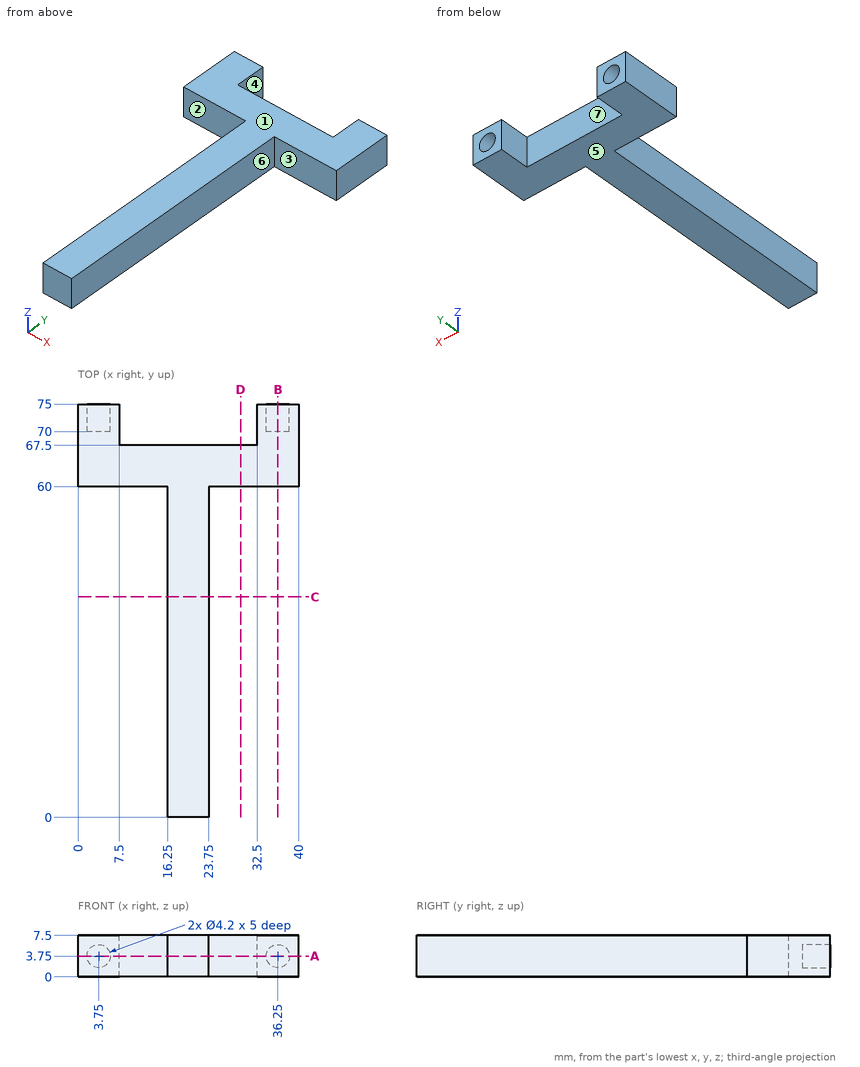
Design review of the part shown in the three views and the two pictorial views. Dimensions are in mm from the part's minimum x, y and z. A direction names the side the tool comes from. Give positions to 0.01 mm unless a question says otherwise; leave off trailing zeros. Loops run counter-clockwise (first coordinate to the right, second up) from the corner with the lowest first, then second, coordinate; pieces in that order, holes last. Notation, with made-up numbers: (-20, 41) -> (1, 41) arc R36 cw to (1, 78) -> close; hole circle Ø3 at (37, 69.25). An arc over 180 degrees is marked (long way). Answer as a JSON object with one key per item and string values. Group by question number.
Q1. Insertion check: pin 1 (4 mm diameter, centred on y = 39.5, z = 3.5, fed in from -X); pin 2 (4 mm diameter, centred on y = 35, z = 5.5, fed in from +X); pin 3 (3 mm diameter, centred on x = 35, z = 4, fed in from -Y). Each pin has a flat end and moves straight along its axis. Give the tip position at first contact, or say it passes through.
Q2. Take a section at D-D (x = 29.5). Write out the cut boundary in (y, z), plus the area to 4 significant figures.
Q3. Take a section at C-C (y = 40). Write out the cut boundary in (x, z).
Q4. Draft analysis for pull direction X (two halves, no side actions). For the marked faces 5, 6 and 7, state which applies: pulls with the +X half, pulls with the -X half, needs draft (parallel to the pull), parting line crosses it, or undercut.
Q5. Take a section at A-A (z = 3.75). Write out the cut boundary in (x, y), plus the area to 4 significant figures.
Q6. Take a section at B-B (x = 36.25). Write out the cut boundary in (y, z).
Q7. Tool access review of the marked faces 1, 2, 3 and 4: name each direction out of +Z, -Z, +X, -X, +Y, -Y from which nothing blocks a thin tool from reaching the whole face with its end or side.
Q8. Wall thickness on line 1 along X through (y, z) = (72.7, 3.75); line 2 along Z through (x, y) = (36, 73); line 3 along X through (y, z) = (71, 3): over which ranges is each line inside the solid? List them lowest first.
Answer below:
{
 "1": {"pin 1": "stops at x = 16.25", "pin 2": "stops at x = 23.75", "pin 3": "stops at y = 60"},
 "2": {"outline": "(60, 0) -> (67.5, 0) -> (67.5, 7.5) -> (60, 7.5) -> close", "area": "56.25 mm2"},
 "3": {"outline": "(16.25, 0) -> (23.75, 0) -> (23.75, 7.5) -> (16.25, 7.5) -> close"},
 "4": {"face 5": "needs draft", "face 6": "pulls with the +X half", "face 7": "undercut"},
 "5": {"outline": "(0, 60) -> (16.25, 60) -> (16.25, 0) -> (23.75, 0) -> (23.75, 60) -> (40, 60) -> (40, 75) -> (38.35, 75) -> (38.35, 70) -> (34.15, 70) -> (34.15, 75) -> (32.5, 75) -> (32.5, 67.5) -> (7.5, 67.5) -> (7.5, 75) -> (5.85, 75) -> (5.85, 70) -> (1.65, 70) -> (1.65, 75) -> (0, 75) -> close", "area": "820.5 mm2"},
 "6": {"outline": "(60, 0) -> (75, 0) -> (75, 1.65) -> (70, 1.65) -> (70, 5.85) -> (75, 5.85) -> (75, 7.5) -> (60, 7.5) -> close"},
 "7": {"face 1": "+Z, +X, -X, +Y, -Y", "face 2": "+Z, -Z, -X, -Y", "face 3": "+Z, -Z, +X, -Y", "face 4": "+Z, -Z, +Y"},
 "8": {"line 1": "x = 0 to 1.65, 5.85 to 7.5, 32.5 to 34.15, 38.35 to 40", "line 2": "z = 0 to 1.66, 5.84 to 7.5", "line 3": "x = 0 to 1.79, 5.71 to 7.5, 32.5 to 34.29, 38.21 to 40"}
}
